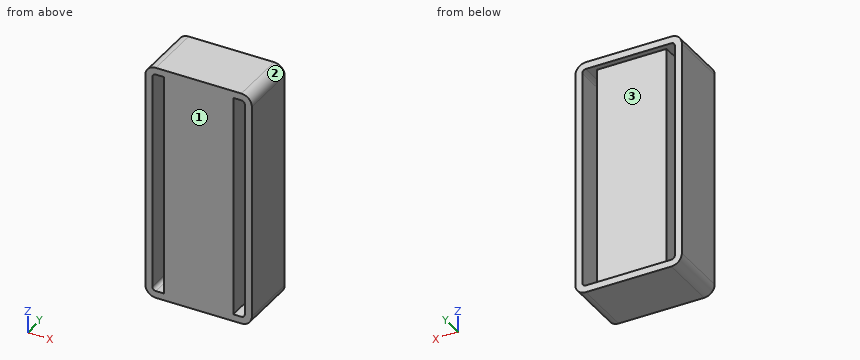
```python
from build123d import *

# Parameters (mm, degrees)
BOSS_EXTRUDE1_DEPTH = 15
BOSS_EXTRUDE2_DEPTH = 1.7


with BuildPart() as part:
    # Sketch1 → Boss-Extrude1 (new body)
    with BuildSketch(Plane(origin=(0, 0, 0), x_dir=(1, 0, 0), z_dir=(0, 1, 0))):
        with BuildLine():
            ThreePointArc((-12.2, 33.9), (-14.321320344, 33.021320344), (-15.2, 30.9))
            Line((-15.2, 30.9), (-15.2, -30.9))
            ThreePointArc((-15.2, -30.9), (-14.321320344, -33.021320344), (-12.2, -33.9))
            Line((-12.2, -33.9), (12.2, -33.9))
            ThreePointArc((12.2, -33.9), (14.321320344, -33.021320344), (15.2, -30.9))
            Line((15.2, -30.9), (15.2, 30.9))
            ThreePointArc((15.2, 30.9), (14.321320344, 33.021320344), (12.2, 33.9))
            Line((12.2, 33.9), (-12.2, 33.9))
        make_face()
        with BuildLine():
            Line((-12.2, 31.9), (-9.9, 31.9))
            Line((-9.9, 31.9), (-9.9, -31.9))
            Line((-9.9, -31.9), (-12.2, -31.9))
            ThreePointArc((-12.2, -31.9), (-12.907106781, -31.607106781), (-13.2, -30.9))
            Line((-13.2, -30.9), (-13.2, 30.9))
            ThreePointArc((-13.2, 30.9), (-12.907106781, 31.607106781), (-12.2, 31.9))
        make_face(mode=Mode.SUBTRACT)
        with BuildLine():
            Line((12.2, -31.9), (9.9, -31.9))
            Line((9.9, -31.9), (9.9, 31.9))
            Line((9.9, 31.9), (12.2, 31.9))
            ThreePointArc((12.2, 31.9), (12.907106781, 31.607106781), (13.2, 30.9))
            Line((13.2, 30.9), (13.2, -30.9))
            ThreePointArc((13.2, -30.9), (12.907106781, -31.607106781), (12.2, -31.9))
        make_face(mode=Mode.SUBTRACT)
    extrude(amount=BOSS_EXTRUDE1_DEPTH)

    # Sketch2 → Boss-Extrude2 (add)
    with BuildSketch(Plane(origin=(0, 15, 0), x_dir=(1, 0, 0), z_dir=(0, 1, 0))):
        with BuildLine():
            Line((12.2, 33.9), (-12.2, 33.9))
            ThreePointArc((-12.2, 33.9), (-14.321320344, 33.021320344), (-15.2, 30.9))
            Line((-15.2, 30.9), (-15.2, -30.9))
            ThreePointArc((-15.2, -30.9), (-14.321320344, -33.021320344), (-12.2, -33.9))
            Line((-12.2, -33.9), (12.2, -33.9))
            ThreePointArc((12.2, -33.9), (14.321320344, -33.021320344), (15.2, -30.9))
            Line((15.2, -30.9), (15.2, 30.9))
            ThreePointArc((15.2, 30.9), (14.321320344, 33.021320344), (12.2, 33.9))
        make_face()
        with BuildLine():
            Line((12.2, 31.9), (-12.2, 31.9))
            ThreePointArc((-12.2, 31.9), (-12.907106781, 31.607106781), (-13.2, 30.9))
            Line((-13.2, 30.9), (-13.2, -30.9))
            ThreePointArc((-13.2, -30.9), (-12.907106781, -31.607106781), (-12.2, -31.9))
            Line((-12.2, -31.9), (12.2, -31.9))
            ThreePointArc((12.2, -31.9), (12.907106781, -31.607106781), (13.2, -30.9))
            Line((13.2, -30.9), (13.2, 30.9))
            ThreePointArc((13.2, 30.9), (12.907106781, 31.607106781), (12.2, 31.9))
        make_face(mode=Mode.SUBTRACT)
    extrude(amount=BOSS_EXTRUDE2_DEPTH)


solid = part.part
```
Source: CAD feature listing. Evaluate the final solid. Frame: model axes, mm. Face numbers are marked on the shaded views. Give positions to 0.01 mm unless a question says otherwise; leave off trailing zeros. Order: outer loops, then holes, each group sorted by start corner. A loop starts at its lowest first (then second) coordinate and runs counter-clockwise, first axis right, second up. Notation, with made-up numbers: (14, -11) -> (68, -11) arc R30 cw to (68, 17) -> close; hole circle Ø2 at (-34, 17). An arc over 180 degrees is marked (long way). Use a Markdown table: item, result.
Q1. Pull-direction query (Z, two-part tool) for the marked faces 1, 2 and 3; classes: +Z half, -Z half, draft (parallel to the pull), parting line (faces both ways), or undercut.
A:
| item | result |
|---|---|
| face 1 | draft |
| face 2 | +Z half |
| face 3 | undercut |
Q2. Material intervals for line 1 (X direction, y = 9.75, z = 8); line 2 (X direction, y = 15.25, z = -14.5); line 3 (Z direction, x = -9.5, y = 16.25), sorted ascending. Write a range as [from, to].
A:
| item | result |
|---|---|
| line 1 | [-15.2, -13.2], [-9.9, 9.9], [13.2, 15.2] |
| line 2 | [-15.2, -13.2], [13.2, 15.2] |
| line 3 | [-33.9, -31.9], [31.9, 33.9] |
Q3. Section B-B (x = 11.5). Return the cut outline in (y, z), and give its area (3 significant figures).
A:
| item | result |
|---|---|
| outline | (0, -33.9) -> (16.7, -33.9) -> (16.7, -31.9) -> (0, -31.9) -> close; (0, 31.9) -> (16.7, 31.9) -> (16.7, 33.9) -> (0, 33.9) -> close |
| area | 66.8 mm^2 |
Q4. First-contact query: P1, Ø10, axis at x = -4.5, z = -22, coming from the +Y side. Flat tip, straight axial feed; report the tip coordinate or a pass-through.
A:
| item | result |
|---|---|
| P1 | y = 15 |
Q5. Section D-D (x = -1). Return the cut outline in (y, z), and give its area (3 significant figures).
A:
| item | result |
|---|---|
| outline | (0, -33.9) -> (16.7, -33.9) -> (16.7, -31.9) -> (15, -31.9) -> (15, 31.9) -> (16.7, 31.9) -> (16.7, 33.9) -> (0, 33.9) -> close |
| area | 1,020 mm^2 |
Q6. Section C-C (y = 2.5). Return the cut outline in (x, z), and give its area (3 significant figures).
A:
| item | result |
|---|---|
| outline | (-15.2, -30.9) arc R3 ccw to (-12.2, -33.9) -> (12.2, -33.9) arc R3 ccw to (15.2, -30.9) -> (15.2, 30.9) arc R3 ccw to (12.2, 33.9) -> (-12.2, 33.9) arc R3 ccw to (-15.2, 30.9) -> close; hole (-13.2, -30.9) arc R1 ccw to (-12.2, -31.9) -> (-9.9, -31.9) -> (-9.9, 31.9) -> (-12.2, 31.9) arc R1 ccw to (-13.2, 30.9) -> close; hole (9.9, -31.9) -> (12.2, -31.9) arc R1 ccw to (13.2, -30.9) -> (13.2, 30.9) arc R1 ccw to (12.2, 31.9) -> (9.9, 31.9) -> close |
| area | 1,630 mm^2 |
Q7. Section A-A (z = 28). Return the cut outline in (x, y).
A:
| item | result |
|---|---|
| outline | (-15.2, 0) -> (-13.2, 0) -> (-13.2, 16.7) -> (-15.2, 16.7) -> close; (-9.9, 0) -> (9.9, 0) -> (9.9, 15) -> (-9.9, 15) -> close; (13.2, 0) -> (15.2, 0) -> (15.2, 16.7) -> (13.2, 16.7) -> close |
